Verification items for the finished model (mm, model axes). A direction names the side the tool comes from. Round coordinates to 2 decimals unless told otherwise and drop trailing zeros. Write each loop counter-clockwise with the first axis right and the second up, starting at its lowest first coordinate (ties: lowest second). Pieces come first, ordered by that corner, then holes. Notation, with made-up numbers: (19, 87) - (62, 87) arc R25 cw to (62, 111) - close; hole circle Ø5 at (77, -21). An arc over 180 degrees is marked (long way). Answer as a JSON object with one key per item and string values.
```python
from build123d import *

# Parameters (mm, degrees)
SKETCH1_W           = 100
SKETCH1_H           = 100
BOSS_EXTRUDE1_DEPTH = 50
SKETCH3_W           = 80
SKETCH3_H           = 30
CUT_EXTRUDE2_DEPTH  = 15
FILLET1_R           = 10
SKETCH4_R           = 10
CUT_EXTRUDE3_DEPTH  = 15
SKETCH5_R           = 10
CUT_EXTRUDE4_DEPTH  = 146.688022843
SKETCH6_W           = 100
SKETCH6_H           = 50
BOSS_EXTRUDE2_DEPTH = 50
FILLET2_R           = 0.1
SKETCH7_R           = 4.224664999
CUT_EXTRUDE5_DEPTH  = 207.155281281
FILLET3_R           = 0.5


with BuildPart() as part:
    # Sketch1 → Boss-Extrude1 (new body)
    with BuildSketch(Plane(origin=(0, 0, 0), x_dir=(1, 0, 0), z_dir=(0, 1, 0))):
        with Locations((50, 50)):
            Rectangle(SKETCH1_W, SKETCH1_H)
    extrude(amount=BOSS_EXTRUDE1_DEPTH)

    # Sketch3 → Cut-Extrude2 (cut)
    with BuildSketch(Plane(origin=(0, 50, 0), x_dir=(1, 0, 0), z_dir=(0, 1, 0))):
        with Locations((50, 25)):
            Rectangle(SKETCH3_W, SKETCH3_H)
    extrude(amount=-CUT_EXTRUDE2_DEPTH, mode=Mode.SUBTRACT)

    # Fillet1
    fillet1_edges = [part.edges().sort_by_distance(p)[0] for p in [
        (10, 42.5, -10),
        (10, 42.5, -40),
        (90, 42.5, -40),
        (90, 42.5, -10),
    ]]
    fillet(fillet1_edges, radius=FILLET1_R)

    # Sketch4 → Cut-Extrude3 (cut)
    with BuildSketch(Plane(origin=(0, 35, 0), x_dir=(1, 0, 0), z_dir=(0, 1, 0))):
        with Locations(Location((25, 25, 0), (0, 0, 270))):
            Circle(SKETCH4_R)
        with Locations(Location((75, 25, 0), (0, 0, 270))):
            Circle(SKETCH4_R)
    extrude(amount=-CUT_EXTRUDE3_DEPTH, mode=Mode.SUBTRACT)

    # Sketch5 → Cut-Extrude4 (cut, through all)
    with BuildSketch(Plane(origin=(0, 35, 0), x_dir=(1, 0, 0), z_dir=(0, 1, 0))):
        with Locations(Location((50, 25, 0), (0, 0, 270))):
            Circle(SKETCH5_R)
    extrude(amount=-CUT_EXTRUDE4_DEPTH, mode=Mode.SUBTRACT)

    # Sketch6 → Boss-Extrude2 (add, symmetric)
    with BuildSketch(Plane.XZ):
        with Locations((50, -125)):
            Rectangle(SKETCH6_W, SKETCH6_H)
    extrude(amount=BOSS_EXTRUDE2_DEPTH, both=True)

    # Fillet2
    fillet2_edges = [part.edges().sort_by_distance(p)[0] for p in [
        (50, 50, -150),
    ]]
    fillet(fillet2_edges, radius=FILLET2_R)

    # Sketch7 → Cut-Extrude5 (cut, through all)
    with BuildSketch(Plane(origin=(0, 50, 0), x_dir=(1, 0, 0), z_dir=(0, 1, 0))):
        with Locations(Location((5.480381348, 62.854130386, 0), (0, 0, 270))):
            Circle(SKETCH7_R)
    extrude(amount=-CUT_EXTRUDE5_DEPTH, mode=Mode.SUBTRACT)

    # Fillet3
    fillet3_edges = [part.edges().sort_by_distance(p)[0] for p in [
        (50, 0, -100),
    ]]
    fillet(fillet3_edges, radius=FILLET3_R)


solid = part.part
```
Q1. Gauge pin test, flat ends, axial feed: P1, Ø23, axis at x = 50, z = -25, coming from the -Y side; P2, Ø15, axis at x = 28, y = -19.5, coming from the +Z side; P3, Ø15, axis at x = 31, z = -24, coming from the +Y side. Record the tip position at first contact, or that the pin passes through.
Geometry check:
{"P1": "stops at y = 0", "P2": "stops at z = -100", "P3": "stops at y = 35"}
Q2. Section check C-C, the plane y = 24. Record the cut outline in (x, z), then the cut area to 3 significant figures.
Geometry check:
{"outline": "(0, -150) - (100, -150) - (100, 0) - (0, 0) - close; hole circle Ø8.45 at (5.48, -62.85); hole circle Ø20 at (25, -25); hole circle Ø20 at (50, -25); hole circle Ø20 at (75, -25)", "area": "14,000 mm2"}
Q3. Set-up check for faces 5 (the flat face through (49, 50, -74)), 6 (the cylindrical face through (13.01, 42.4, -37.15)): record each of +Z, -Z, +X, -X, +Y, -Y from which the full face is reachable in a straight line by a thin tool's end or side.
Geometry check:
{"face 5": "+Z, -Z, +X, -X, +Y", "face 6": "+Y"}
Q4. Section check D-D, the plane x = 62.5. Record the cut outline in (y, z), then the cut area to 3 significant figures.
Geometry check:
{"outline": "(-50, -150) - (49.9, -150) arc R0.1 ccw to (50, -149.9) - (50, -40) - (35, -40) - (35, -10) - (50, -10) - (50, 0) - (0, 0) - (0, -99.5) arc R0.5 cw to (-0.5, -100) - (-50, -100) - close", "area": "9,550 mm2"}
Q5. Section check A-A, the plane x = 50. Record the cut outline in (y, z).
Geometry check:
{"outline": "(-50, -150) - (49.9, -150) arc R0.1 ccw to (50, -149.9) - (50, -40) - (35, -40) - (35, -35) - (0, -35) - (0, -99.5) arc R0.5 cw to (-0.5, -100) - (-50, -100) - close; (0, -15) - (35, -15) - (35, -10) - (50, -10) - (50, 0) - (0, 0) - close"}
Q6. Release check for a two-part mould opening along X. For faces 1 (the flat face through (0, 10, -93)), 2 (the flat face through (100, 10, -93)), 3 (the flat face through (49, -26, -100)), 4 (the cylindrical face through (28, 27.6, -15.46)) record: released by +X, released by -X, zero draft, split by the parting line, or undercut.
Geometry check:
{"face 1": "released by -X", "face 2": "released by +X", "face 3": "zero draft", "face 4": "undercut"}
Q7. Material ranges on line 1 along X through (y, z) = (27, -25); line 2 along X through (y, z) = (13, -25); line 3 along Y through (x, z) = (43.5, -40.5), recorded low to high. Write a range as [from, to].
Geometry check:
{"line 1": "x = [0, 15], [35, 40], [60, 65], [85, 100]", "line 2": "x = [0, 40], [60, 100]", "line 3": "y = [0, 50]"}
Q8. Section check B-B, the plane z = -25. Record the cut outline in (x, y).
Geometry check:
{"outline": "(0, 0) - (40, 0) - (40, 35) - (35, 35) - (35, 20) - (15, 20) - (15, 35) - (10, 35) - (10, 50) - (0, 50) - close; (60, 0) - (100, 0) - (100, 50) - (90, 50) - (90, 35) - (85, 35) - (85, 20) - (65, 20) - (65, 35) - (60, 35) - close"}
